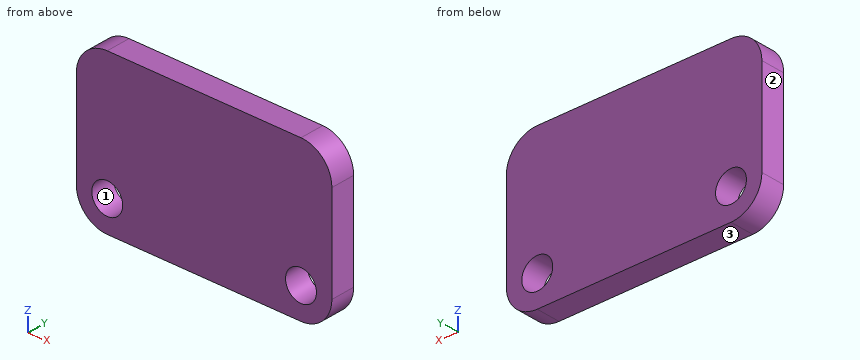
```python
from build123d import *

# Parameters (mm, degrees)
SKETCH1_W           = 21
SKETCH1_H           = 13
BOSS_EXTRUDE1_DEPTH = 2
SKETCH2_R           = 1.27
CUT_EXTRUDE1_DEPTH  = 3
FILLET1_R           = 2.54


with BuildPart() as part:
    # Sketch1 → Boss-Extrude1 (new body)
    with BuildSketch(Plane(origin=(0, 0, 0), x_dir=(1, 0, 0), z_dir=(0, 1, 0))):
        with Locations((10.5, 6.5)):
            Rectangle(SKETCH1_W, SKETCH1_H)
    extrude(amount=BOSS_EXTRUDE1_DEPTH)

    # Sketch2 → Cut-Extrude1 (cut, through all)
    with BuildSketch(Plane(origin=(0, 2, 0), x_dir=(1, 0, 0), z_dir=(0, 1, 0))):
        with Locations((2.54, 10.46)):
            Circle(SKETCH2_R)
        with Locations((18.46, 10.46)):
            Circle(SKETCH2_R)
    extrude(amount=-CUT_EXTRUDE1_DEPTH, mode=Mode.SUBTRACT)

    # Fillet1
    fillet1_edges = [part.edges().sort_by_distance(p)[0] for p in [
        (0, 1, -13),
        (21, 1, -13),
        (21, 1, 0),
        (0, 1, 0),
    ]]
    fillet(fillet1_edges, radius=FILLET1_R)


solid = part.part
```
Could you check a few things on this model? Use its own coordinates, in mm. Face numbers are marked on the shaded views. Give positions to 0.01 mm unless a question says otherwise; leave off trailing zeros. Order: outer loops, then holes, each group sorted by start corner. A loop starts at its lowest first (then second) coordinate and runs counter-clockwise, first axis right, second up.
Q1. Suppose I cut it at A-A, the plane y = 0.3. Write out the boundary of the cut face in (x, z), and give its area (3 significant figures).
Q2. If I drill on line 1 along X through (y, z) = (0.85, -10.46); line 2 along Z through (x, y) = (18.46, 0.75); line 3 along X through (y, z) = (0.45, -11.25), over which ranges is the centre line in solid material (lowest first)?
Q3. Suppose I cut it at B-B, the plane x = 18.75. Write out the boundary of the cut face in (y, z), and give its area (3 significant figures).
Q4. We'd pull the mould along Z, two halves only. Please class the marked faces 1, 2 and 3: +Z half, -Z half, draft (parallel to the pull), parting line (faces both ways), or undercut.
Solution:
1. outline: (0, -10.46) arc R2.54 ccw to (2.54, -13) - (18.46, -13) arc R2.54 ccw to (21, -10.46) - (21, -2.54) arc R2.54 ccw to (18.46, 0) - (2.54, 0) arc R2.54 ccw to (0, -2.54) - close; hole circle Ø2.54 at (2.54, -10.46); hole circle Ø2.54 at (18.46, -10.46)
1. area: 257 mm2
2. line 1: x = 0 to 1.27, 3.81 to 17.19, 19.73 to 21
2. line 2: z = -13 to -11.73, -9.19 to 0
2. line 3: x = 0.13 to 1.55, 3.53 to 17.47, 19.45 to 20.87
3. outline: (0, -12.98) - (2, -12.98) - (2, -11.7) - (0, -11.7) - close; (0, -9.22) - (2, -9.22) - (2, -0.02) - (0, -0.02) - close
3. area: 21.0 mm2
4. face 1: undercut
4. face 2: draft
4. face 3: -Z half
